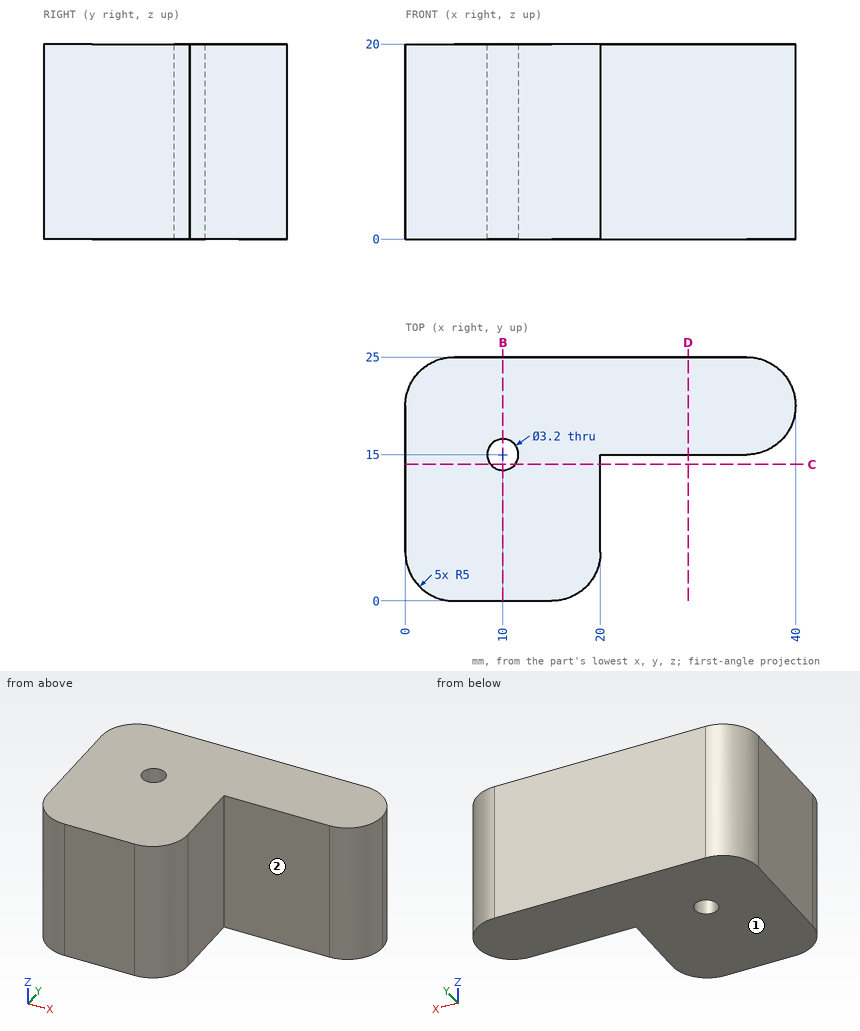
Study the drawing (mm; zero at the part's minimum x, y, z) and answer. A direction names the side the tool comes from. Give positions to 0.01 mm unless a question says otherwise; leave off trailing zeros. Write each loop counter-clockwise with the first axis right and the second up, starting at its lowest first coordinate (ties: lowest second). Pieces come first, ordered by that corner, then holes. Notation, with made-up numbers: (-20.75, 66) - (27.25, 66) arc R21 cw to (27.25, 70) - close; hole circle Ø3 at (-23.75, -31.5). An arc over 180 degrees is marked (long way). One line per question, with ' | ' between items. Start each with the question number.
1. Section B-B, the plane x = 10 is taken. Determine the outline of the cut face in (y, z).
2. Given P1, Ø12, axis at y = 21.5, z = 11.5, coming from the -X side; P2, Ø12, axis at x = 31, z = 14, coming from the -Y side; P3, Ø12, axis at y = 5, z = 17.5, coming from the +X side, each flat-ended and moving along its own axis, determine where each tip first touches the part or whether it passes through.
3. Section D-D, the plane x = 29 is taken. Determine the outline of the cut face in (y, z), then the cut area to 3 significant figures.
4. For the marked faces 1 and 2, determine the directions among +Z, -Z, +X, -X, +Y, -Y from which every point of the face is accessible in a straight line to the end or side of a thin tool.
5. Section C-C, the plane y = 14 is taken. Determine the outline of the cut face in (x, z), then the cut area to 3 significant figures.
6. Straight lines are drawn through the part: line 1 (Y direction, x = 10, z = 8); line 2 (X direction, y = 11.75, z = 7); line 3 (Y direction, x = 22, z = 13.5). For each, find the intervals that lie inside material, in ascending order.
Result:
1) outline: (0, 0) - (13.4, 0) - (13.4, 20) - (0, 20) - close; (16.6, 0) - (25, 0) - (25, 20) - (16.6, 20) - close
2) P1: stops at x = 0 | P2: stops at y = 15 | P3: stops at x = 20
3) outline: (15, 0) - (25, 0) - (25, 20) - (15, 20) - close | area: 200 mm2
4) face 1: -Z, +X, -X, +Y, -Y | face 2: +Z, -Z, +X, -Y
5) outline: (0, 0) - (8.75, 0) - (8.75, 20) - (0, 20) - close; (11.25, 0) - (20, 0) - (20, 20) - (11.25, 20) - close | area: 350 mm2
6) line 1: y = 0 to 13.4, 16.6 to 25 | line 2: x = 0 to 20 | line 3: y = 15 to 25
